```python
from build123d import *

# Parameters (mm, degrees)
SKETCH1_W           = 24
SKETCH1_H           = 25
BOSS_EXTRUDE1_DEPTH = 8
SKETCH2_R           = 4
CUT_EXTRUDE1_DEPTH  = 29.217902119
SKETCH3_R           = 2.6
CUT_EXTRUDE2_DEPTH  = 20.085334684
FILLET1_R           = 3
FILLET2_R           = 5
CUT_EXTRUDE3_DEPTH  = 4.5


with BuildPart() as part:
    # Sketch1 → Boss-Extrude1 (new body)
    with BuildSketch(Plane(origin=(0, 0, 0), x_dir=(1, 0, 0), z_dir=(0, 1, 0))):
        Rectangle(SKETCH1_W, SKETCH1_H)
    extrude(amount=BOSS_EXTRUDE1_DEPTH)

    # Sketch2 → Cut-Extrude1 (cut, through all)
    with BuildSketch(Plane.ZY.offset(12)):
        Circle(SKETCH2_R)
    extrude(amount=-CUT_EXTRUDE1_DEPTH, mode=Mode.SUBTRACT)

    # Sketch3 → Cut-Extrude2 (cut, through all)
    with BuildSketch(Plane.XZ):
        with Locations(Location((-6, -7, 0), (0, 0, 270))):
            Circle(SKETCH3_R)
        with Locations(Location((6, 7, 0), (0, 0, 270))):
            Circle(SKETCH3_R)
    extrude(amount=-CUT_EXTRUDE2_DEPTH, mode=Mode.SUBTRACT)

    # Fillet1
    # the kernel refuses this fillet: 3 mm, written as the material it takes off along each edge
    with BuildSketch(Plane(origin=(19.5, 8, 12.5), x_dir=(0, 0, -1), z_dir=(-1, 0, 0))) as fillet1_piece_1:
        with BuildLine():
            CenterArc((FILLET1_R, FILLET1_R), FILLET1_R, 180, 90)
            Line((0, FILLET1_R), (0, 0))
            Line((0, 0), (FILLET1_R, 0))
        make_face()
    extrude(amount=39, mode=Mode.SUBTRACT)
    with BuildSketch(Plane(origin=(12, 8, -20), x_dir=(0, -1, 0), z_dir=(0, 0, 1))) as fillet1_piece_2:
        with BuildLine():
            CenterArc((FILLET1_R, -FILLET1_R), FILLET1_R, 90, 90)
            Line((0, -FILLET1_R), (0, 0))
            Line((0, 0), (FILLET1_R, 0))
        make_face()
    extrude(amount=40, mode=Mode.SUBTRACT)
    with BuildSketch(Plane(origin=(-19.5, 8, -12.5), x_dir=(0, -1, 0), z_dir=(1, 0, 0))) as fillet1_piece_3:
        with BuildLine():
            CenterArc((FILLET1_R, -FILLET1_R), FILLET1_R, 90, 90)
            Line((0, -FILLET1_R), (0, 0))
            Line((0, 0), (FILLET1_R, 0))
        make_face()
    extrude(amount=39, mode=Mode.SUBTRACT)

    # Fillet2
    # the kernel refuses this fillet: 5 mm, written as the material it takes off along each edge
    with BuildSketch(Plane(origin=(7, 8, 7.5), x_dir=(0, 0, 1), z_dir=(-1, 0, 0))) as fillet2_piece_1:
        with BuildLine():
            CenterArc((2, -3), 3, 0, 90)
            Line((5, -3), (5, 0))
            Line((5, 0), (2, 0))
        make_face()
    revolve(axis=Axis((7, 8, 7.5), (0, 1, 0)), revolution_arc=90, mode=Mode.SUBTRACT)
    with BuildSketch(Plane(origin=(7, 8, -7.5), x_dir=(1, 0, 0), z_dir=(0, 0, 1))) as fillet2_piece_2:
        with BuildLine():
            CenterArc((2, -3), 3, 0, 90)
            Line((5, -3), (5, 0))
            Line((5, 0), (2, 0))
        make_face()
    revolve(axis=Axis((7, 8, -7.5), (0, 1, 0)), revolution_arc=90, mode=Mode.SUBTRACT)
    with BuildSketch(Plane(origin=(12, -12.5, -12.5), x_dir=(-1, 0, 0), z_dir=(0, 1, 0)), Plane(origin=(12, -12.5, 12.5), x_dir=(0, 0, -1), z_dir=(0, 1, 0))) as fillet2_piece_3:
        with BuildLine():
            CenterArc((FILLET2_R, FILLET2_R), FILLET2_R, 180, 90)
            Line((0, FILLET2_R), (0, 0))
            Line((0, 0), (FILLET2_R, 0))
        make_face()
    extrude(amount=20.5, mode=Mode.SUBTRACT)

    # Sketch4 → Cut-Extrude3 (cut)
    with BuildSketch(Plane(origin=(0, 8, 0), x_dir=(1, 0, 0), z_dir=(0, 1, 0))):
        Polygon((6, -11.792007234), (10.15, -9.396003617), (10.15, -4.603996383), (6, -2.207992766), (1.85, -4.603996383), (1.85, -9.396003617), align=None)
        Polygon((-6.063761716, 2.208416986), (-1.882248244, 4.548989227), (-1.818486528, 9.340572241), (-5.936238284, 11.791583014), (-10.117751756, 9.451010773), (-10.181513472, 4.659427759), align=None)
    extrude(amount=-CUT_EXTRUDE3_DEPTH, mode=Mode.SUBTRACT)


solid = part.part
```
Geometry: final body of the model. Coordinates: model frame, mm. A direction names the side the tool comes from. Round coordinates to 2 decimals unless told otherwise and drop trailing zeros. Loops run counter-clockwise (first coordinate to the right, second up) from the corner with the lowest first, then second, coordinate; pieces in that order, holes last. Notation, with made-up numbers: (41, -12.75) -> (97, -12.75) arc R19 cw to (97, 22.25) -> close; hole circle Ø3 at (24.25, -19). An arc over 180 degrees is marked (long way). Use one line per item in the form item = value.
Item 1: Cut plane B-B on y = 2. Output: boundary loops of the cut face in (x, z), then the cut area to 3 significant figures.
Evaluation:
outline = (-12, -12.5) -> (7, -12.5) arc R5 ccw to (12, -7.5) -> (12, -3.46) -> (-12, -3.46) -> close; (-12, 3.46) -> (12, 3.46) -> (12, 7.5) arc R5 ccw to (7, 12.5) -> (-12, 12.5) -> close; hole circle Ø5.2 at (-6, -7); hole circle Ø5.2 at (6, 7)
area = 381 mm2
Item 2: Cut plane D-D on x = -7. Output: boundary loops of the cut face in (y, z).
Evaluation:
outline = (0, -12.5) -> (5, -12.5) arc R3 ccw to (7.47, -11.2) -> (3.5, -11.2) -> (3.5, -9.4) -> (0, -9.4) -> close; (0, -4.6) -> (3.5, -4.6) -> (3.5, -2.77) -> (8, -2.77) -> (8, 9.5) arc R3 ccw to (5, 12.5) -> (0, 12.5) -> (0, 4) arc R4 cw to (0, -4) -> close
Item 3: Contact query for flat-ended pins moving along their axis: pin 1 Ø6.5 at (x, z) = (7.5, 8.5) entering from +Y; pin 2 Ø2.5 at (x, z) = (-6, -5.5) entering from +Y. Output: stop coordinate, or through.
Evaluation:
pin_1 = 7.77
pin_2 = 3.5
Item 4: Cut plane A-A on z = 7. Output: boundary loops of the cut face in (x, y).
Evaluation:
outline = (-12, 0) -> (3.4, 0) -> (3.4, 3.5) -> (1.85, 3.5) -> (1.85, 8) -> (-12, 8) -> close; (8.6, 0) -> (12, 0) -> (12, 5) arc R3 ccw to (10.15, 7.77) -> (10.15, 3.5) -> (8.6, 3.5) -> close
Item 5: Material intervals for probe 1 along X at (y, z) = (1.35, -7); probe 2 along X at (y, z) = (1.55, 7); probe 3 along Z at (x, y) = (5.5, 3.25), sorted ascending.
Evaluation:
probe_1 = -12 to -8.6, -3.4 to 12
probe_2 = -12 to 3.4, 8.6 to 12
probe_3 = -12.5 to -2.33, 2.33 to 4.45, 9.55 to 12.5
Item 6: Cut plane C-C on y = 4.5. Output: boundary loops of the cut face in (x, z), then the cut area to 3 significant figures.
Evaluation:
outline = (-12, -12.5) -> (7, -12.5) arc R5 ccw to (12, -7.5) -> (12, 7.5) arc R5 ccw to (7, 12.5) -> (-12, 12.5) -> close; hole (-10.18, -4.66) -> (-10.12, -9.45) -> (-5.94, -11.79) -> (-1.82, -9.34) -> (-1.88, -4.55) -> (-6.06, -2.21) -> close; hole (1.85, 4.6) -> (6, 2.21) -> (10.15, 4.6) -> (10.15, 9.4) -> (6, 11.79) -> (1.85, 9.4) -> close
area = 470 mm2
Item 7: Access query for faces 5 (the flat face through (-3, 2, -12.5)), 6 (the flat face through (-7.998, 5.781, -10.638)). Directions: +Z, -Z, +X, -X, +Y, -Y. A direction counts if a zero-diameter tool reaches every point of the face in a straight line with its end or side. Return the directions, or none.
Evaluation:
face_5 = -Z, +X, -X, +Y, -Y
face_6 = +Y
Item 8: Draft query along X for faces 1 (the cylindrical face through (0, 4, 0)), 2 (the flat face through (10.15, 6, 7)), 3 (the cylindrical face through (-5.22, 1.73, -9.48)), 4 (the flat face through (12, 4.7, 0.1)). Return one class per face: released by +X, released by -X, zero draft, split by the parting line, or undercut.
Evaluation:
face_1 = zero draft
face_2 = undercut
face_3 = undercut
face_4 = released by +X
